Here's how the part is built. I have some questions about the finished solid (model axes, mm). A direction names the side the tool comes from. Round coordinates to 2 decimals unless told otherwise and drop trailing zeros. Order: outer loops, then holes, each group sorted by start corner. A loop starts at its lowest first (then second) coordinate and runs counter-clockwise, first axis right, second up. Notation, with made-up numbers: (-30, 70.25) -> (-5, 70.25) arc R29 ccw to (-5, 90.25) -> close; hole circle Ø2 at (-10, -8.75). An arc over 180 degrees is marked (long way). Use a Markdown table: item, result. Add a question column.
(1) Thinking about a two-plate mould opening in Y: for faces 5 (the face through (6.084, 11.666, -5.983)), 6 (the face through (6, 50, -49)), 7 (the face through (37, 25, -59)), 8 (the face through (6.08, 7.35, -86.55)), which applies, pulls with the +Y half, pulls with the -Y half, needs draft (parallel to the pull), parting line crosses it, or undercut?
(2) I want a section at C-C, the plane z = -90. Please give me the cut outline in (x, y).
(3) On a 3-axis mill with a long thin cutter (end or side, diameter ignored), from which of +Z, -Z, +X, -X, +Y, -Y can I reach the whole of each face in a straight line? I mean faces 1 (the face through (18, 21, -26)), 2 (the face through (12, 36, -38)), 3 (the face through (34, 15, -46.025)), 4 (the face through (18, 21, -75)). Say none if no direction works.
(4) I want a section at B-B, the plane x = 20.5. Please give me the cut outline in (y, z).
(5) If I drill on probe 1 along Y at (x, z) = (8.75, -90); probe 2 along X at (y, z) = (5, -6); probe 3 along Y at (x, z) = (15, -34.5), over which ranges is the centre line in solid material (lowest first)?
(6) I want a section at A-A, the plane x = 9. Please give me the cut outline in (y, z), then the cut area to 3 significant figures.
(7) I'm going to push flat-ended pins straight in: P1, Ø17, axis at x = 21, z = -22.5, coming from the +Y side; P2, Ø1.5, axis at x = 35.5, y = 16.5, coming from the +Z side; P3, Ø2, axis at y = 41.5, z = -84.5, coming from the +X side; P4, Ø2, axis at x = 25, z = -81.5, coming from the +Y side. Where does each tip first touch, or does it pass through?
(8) I want a section at D-D, the plane y = 41. Please give me the cut outline in (x, z), then the cut area to 3 significant figures.
from build123d import *

# Parameters (mm, degrees)
SKETCH_1_W               = 100
SKETCH_1_H               = 50
EXTRUDE_1_DEPTH          = 12
SKETCH_2_R               = 15
SKETCH_2_R_2             = 7.5
EXTRUDE_3_DEPTH          = 25
EXTRUDE_20_DEPTH         = 4
SKETCH_7_R               = 7.5
CUT_EXTRUDE_2_DEPTH      = 115.564392374
CUT_EXTRUDE_4_DEPTH      = 110.517121949
CUT_EXTRUDE_4_DEPTH_BACK = 110.517121949
CUT_EXTRUDE_5_DEPTH      = 110.517121949
CUT_EXTRUDE_5_DEPTH_BACK = 110.517121949
SKETCH_9_R               = 4
SKETCH_10_R              = 4.349058231
CUT_EXTRUDE_6_DEPTH      = 115.564392396


with BuildPart() as part:
    # 草图1 → 凸台-拉伸1 (new body)
    with BuildSketch(Plane(origin=(0, 0, 0), x_dir=(0, 0, -1), z_dir=(1, 0, 0))):
        with Locations((50, 25)):
            Rectangle(SKETCH_1_W, SKETCH_1_H)
    extrude(amount=EXTRUDE_1_DEPTH)

    # 草图2 → 凸台-拉伸3 (add)
    with BuildSketch(Plane(origin=(12, 0, 0), x_dir=(0, 0, -1), z_dir=(1, 0, 0))):
        with Locations((50.025247728, 25)):
            Circle(SKETCH_2_R)
        with Locations((50.025247728, 25)):
            Circle(SKETCH_2_R_2, mode=Mode.SUBTRACT)
    extrude(amount=EXTRUDE_3_DEPTH)

    # 草图6 → 凸台-拉伸20 (add, symmetric)
    with BuildSketch(Plane(origin=(0, 25, 0), x_dir=(1, 0, 0), z_dir=(0, 1, 0))):
        Polygon((11.607924721, 61.899802302), (11.974710876, 100), (34.498075292, 61.899802302), align=None)
        Polygon((11.607924721, 38.150693154), (34.498075292, 38.150693154), (11.974710876, 0.050495456), align=None)
    extrude(amount=EXTRUDE_20_DEPTH, both=True)

    # 草图7 → 切除-拉伸2 (cut, through all)
    with BuildSketch(Plane(origin=(12, 0, 0), x_dir=(0, 0, -1), z_dir=(1, 0, 0))):
        with Locations((50.025247728, 25)):
            Circle(SKETCH_7_R)
    extrude(amount=-CUT_EXTRUDE_2_DEPTH, mode=Mode.SUBTRACT)

    # 草图8 → 切除-拉伸4 (cut, two sides: drawn at the far end of the back side and taken through both)
    with BuildSketch(Plane(origin=(0, 25, 0), x_dir=(1, 0, 0), z_dir=(0, 1, 0)).offset(-CUT_EXTRUDE_4_DEPTH_BACK)):
        Polygon((37, 54.025247728), (32, 54.025247728), (32, 46.025247728), (37, 46.025247728), (37, 50.025247728), align=None)
    extrude(amount=CUT_EXTRUDE_4_DEPTH + CUT_EXTRUDE_4_DEPTH_BACK, mode=Mode.SUBTRACT)

    # 草图9 → 切除-拉伸5 (cut, two sides: drawn at the far end of the back side and taken through both)
    with BuildSketch(Plane(origin=(0, 25, 0), x_dir=(1, 0, 0), z_dir=(0, 1, 0)).offset(-CUT_EXTRUDE_5_DEPTH_BACK)):
        with Locations(Location((22, 50.007690545, 0), (0, 0, 270))):
            Circle(SKETCH_9_R)
    extrude(amount=CUT_EXTRUDE_5_DEPTH + CUT_EXTRUDE_5_DEPTH_BACK, mode=Mode.SUBTRACT)

    # 草图10 → 切除-拉伸6 (cut, through all)
    with BuildSketch(Plane(origin=(12, 0, 0), x_dir=(0, 0, -1), z_dir=(1, 0, 0))):
        with Locations((10, 40)):
            Circle(SKETCH_10_R)
        with Locations(Location((10, 10, 0), (0, 0, 180))):
            Circle(SKETCH_10_R)
        with Locations((90, 10)):
            Circle(SKETCH_10_R)
        with Locations(Location((90, 40, 0), (0, 0, 180))):
            Circle(SKETCH_10_R)
    extrude(amount=-CUT_EXTRUDE_6_DEPTH, mode=Mode.SUBTRACT)


solid = part.part
Taken from the geometry:
| question | item | result |
|---|---|---|
| 1 | face 5 | undercut |
| 1 | face 6 | pulls with the +Y half |
| 1 | face 7 | needs draft |
| 1 | face 8 | undercut |
| 2 | outline | (0, 0) -> (12, 0) -> (12, 5.65) -> (0, 5.65) -> close; (0, 14.35) -> (12, 14.35) -> (12, 21) -> (17.89, 21) -> (17.89, 29) -> (12, 29) -> (12, 35.65) -> (0, 35.65) -> close; (0, 44.35) -> (12, 44.35) -> (12, 50) -> (0, 50) -> close |
| 3 | face 1 | +Z, +X, -Y |
| 3 | face 2 | +X |
| 3 | face 3 | +X, +Y, -Y |
| 3 | face 4 | -Z, +X, -Y |
| 4 | outline | (10.46, -53.72) arc R15 ccw to (21, -64.48) -> (21, -85.58) -> (29, -85.58) -> (29, -64.48) arc R15 ccw to (39.54, -53.72) -> (31.53, -53.72) arc R7.5 cw to (18.47, -53.72) -> close; (10.47, -46.3) -> (18.49, -46.3) arc R7.5 cw to (31.51, -46.3) -> (39.53, -46.3) arc R15 ccw to (29, -35.57) -> (29, -14.47) -> (21, -14.47) -> (21, -35.57) arc R15 ccw to start |
| 5 | probe 1 | y = 0 to 5.65, 14.35 to 35.65, 44.35 to 50 |
| 5 | probe 2 | x = 0 to 12 |
| 5 | probe 3 | y = 21 to 29 |
| 6 | outline | (0, -100) -> (50, -100) -> (50, 0) -> (0, 0) -> close; hole circle Ø8.7 at (10, -90); hole circle Ø8.7 at (10, -10); hole circle Ø15 at (25, -50.03); hole circle Ø8.7 at (40, -90); hole circle Ø8.7 at (40, -10) |
| 6 | area | 4,590 mm2 |
| 7 | P1 | stops at y = 29 |
| 7 | P2 | stops at z = -37.18 |
| 7 | P3 | stops at x = 12 |
| 7 | P4 | passes through |
| 8 | outline | (0, -100) -> (12, -100) -> (12, -94.23) -> (0, -94.23) -> close; (0, -85.77) -> (12, -85.77) -> (12, -14.23) -> (0, -14.23) -> close; (0, -5.77) -> (12, -5.77) -> (12, 0) -> (0, 0) -> close |
| 8 | area | 997 mm2 |
